Input: part model. Units: mm. Frame: model coordinates. A direction names the side the tool comes from. Give positions to 0.01 mm unless a question says otherwise; leave off trailing zeros. Order: outer loops, then holes, each group sorted by start corner. A loop starts at its lowest first (then second) coordinate and runs counter-clockwise, first axis right, second up. Notation, with made-up numbers: M 22,66 L 74,66 A25 cw 74,99 Z; hole C 73.25,-27.75 d8. An arc over 180 degrees is marked long. Use a Markdown table: item, result.
from build123d import *

# Parameters (mm, degrees)
SKETCH1_R           = 30
BOSS_EXTRUDE1_DEPTH = 25


with BuildPart() as part:
    # Sketch1 → Boss-Extrude1 (new body)
    with BuildSketch(Plane(origin=(0, 0, 0), x_dir=(1, 0, 0), z_dir=(0, 1, 0))):
        with BuildLine():
            Line((73, 18.485014011), (73, -18.485014011))
            ThreePointArc((73, -18.485014011), (98.171988791, -34.2), (108, -62.2))
            Line((108, -62.2), (108, -107))
            Line((108, -107), (63.2, -107))
            ThreePointArc((63.2, -107), (28.924287458, -91.048146036), (19.057555316, -54.552479005))
            ThreePointArc((19.057555316, -54.552479005), (15.86461811, -44.166949194), (5.59587046, -40.616329645))
            ThreePointArc((5.59587046, -40.616329645), (0, -41), (-5.59587046, -40.616329645))
            ThreePointArc((-5.59587046, -40.616329645), (-15.86461811, -44.166949194), (-19.057555316, -54.552479005))
            ThreePointArc((-19.057555316, -54.552479005), (-28.924287458, -91.048146036), (-63.2, -107))
            Line((-63.2, -107), (-108, -107))
            Line((-108, -107), (-108, -62.2))
            ThreePointArc((-108, -62.2), (-98.171988791, -34.2), (-73, -18.485014011))
            Line((-73, -18.485014011), (-73, 18.485014011))
            ThreePointArc((-73, 18.485014011), (-98.171988791, 34.2), (-108, 62.2))
            Line((-108, 62.2), (-108, 107))
            Line((-108, 107), (-63.2, 107))
            ThreePointArc((-63.2, 107), (-28.924287458, 91.048146036), (-19.057555316, 54.552479005))
            ThreePointArc((-19.057555316, 54.552479005), (-15.86461811, 44.166949194), (-5.59587046, 40.616329645))
            ThreePointArc((-5.59587046, 40.616329645), (0, 41), (5.59587046, 40.616329645))
            ThreePointArc((5.59587046, 40.616329645), (15.86461811, 44.166949194), (19.057555316, 54.552479005))
            ThreePointArc((19.057555316, 54.552479005), (28.924287458, 91.048146036), (63.2, 107))
            Line((63.2, 107), (108, 107))
            Line((108, 107), (108, 62.2))
            ThreePointArc((108, 62.2), (98.171988791, 34.2), (73, 18.485014011))
        make_face()
        with Locations(Location((0, 0, 0), (0, 0, 270))):
            Circle(SKETCH1_R, mode=Mode.SUBTRACT)
        with BuildLine():
            Line((86.274940548, 85.274940548), (86.274940548, 62.2))
            ThreePointArc((86.274940548, 62.2), (46.883553063, 45.883553063), (63.2, 85.274940548))
            Line((63.2, 85.274940548), (86.274940548, 85.274940548))
        make_face(mode=Mode.SUBTRACT)
        with BuildLine():
            Line((86.274940548, -85.274940548), (86.274940548, -62.2))
            ThreePointArc((86.274940548, -62.2), (46.883553063, -45.883553063), (63.2, -85.274940548))
            Line((63.2, -85.274940548), (86.274940548, -85.274940548))
        make_face(mode=Mode.SUBTRACT)
        with BuildLine():
            Line((-86.274940548, -85.274940548), (-86.274940548, -62.2))
            ThreePointArc((-86.274940548, -62.2), (-46.883553063, -45.883553063), (-63.2, -85.274940548))
            Line((-63.2, -85.274940548), (-86.274940548, -85.274940548))
        make_face(mode=Mode.SUBTRACT)
        with BuildLine():
            Line((-63.2, 85.274940548), (-86.274940548, 85.274940548))
            Line((-86.274940548, 85.274940548), (-86.274940548, 62.2))
            ThreePointArc((-86.274940548, 62.2), (-46.883553063, 45.883553063), (-63.2, 85.274940548))
        make_face(mode=Mode.SUBTRACT)
    extrude(amount=BOSS_EXTRUDE1_DEPTH)


solid = part.part
1) Cut plane A-A on x = 0. Return loops of the section in (y, z), and give its area (3 significant figures).
Response values:
| item | result |
|---|---|
| outline | M 0,-41 L 25,-41 L 25,-30 L 0,-30 Z; M 0,30 L 25,30 L 25,41 L 0,41 Z |
| area | 550 mm² |
2) Cut plane B-B on z = 0. Return loops of the section in (x, y).
Response values:
| item | result |
|---|---|
| outline | M -73,0 L -30,0 L -30,25 L -73,25 Z; M 30,0 L 73,0 L 73,25 L 30,25 Z |
3) Cut plane D-D on x = 76. Return loops of the section in (y, z), and give its area (3 significant figures).
Response values:
| item | result |
|---|---|
| outline | M 0,-107 L 25,-107 L 25,-85.27 L 0,-85.27 Z; M 0,-43 L 25,-43 L 25,-19.27 L 0,-19.27 Z; M 0,19.27 L 25,19.27 L 25,43 L 0,43 Z; M 0,85.27 L 25,85.27 L 25,107 L 0,107 Z |
| area | 2,270 mm² |
4) Mould query, pull axis X, two halves, no side actions, for faces 1 (the face through (98.435, 12.325, -34.532)), 2 (the face through (-108, 12, -84)), 3 (the face through (-86.275, 12, -74)), 4 (the face through (85, 12, -107)). Classes: released by +X, released by -X, zero draft, split by the parting line, or undercut.
Response values:
| item | result |
|---|---|
| face 1 | released by +X |
| face 2 | released by -X |
| face 3 | undercut |
| face 4 | zero draft |
5) Reachability of faces 5 (the face through (-73, 12, 0)), 6 (the face through (-86.275, 12, 74)), 7 (the face through (-108, 12, 85)) from +Z, -Z, +X, -X, +Y, -Y: full face, straight path, thin tool, end or side. Return the list, or none.
Response values:
| item | result |
|---|---|
| face 5 | -X, +Y, -Y |
| face 6 | +Y, -Y |
| face 7 | +Z, -Z, -X, +Y, -Y |
6) Cut plane C-C on z = -76. Return loops of the section in (x, y).
Response values:
| item | result |
|---|---|
| outline | M -108,0 L -86.27,0 L -86.27,25 L -108,25 Z; M -44.71,0 L -20.58,0 L -20.58,25 L -44.71,25 Z; M 20.58,0 L 44.71,0 L 44.71,25 L 20.58,25 Z; M 86.27,0 L 108,0 L 108,25 L 86.27,25 Z |
7) First-contact query: pin 1 Ø1 at (y, z) = (5.5, 49) entering from -X; pin 2 Ø1 at (x, y) = (46.5, 7.5) entering from +Z; pin 3 Ø2 at (x, z) = (-36.5, 34) entering from -Y; pin 4 Ø7.5 at (y, z) = (6.5, 1) entering from -X. Flat tips, straight axial feed; report the tip coordinate or a pass-through.
Response values:
| item | result |
|---|---|
| pin 1 | stops at x = -106.16 |
| pin 2 | stops at z = 103.97 |
| pin 3 | stops at y = 0 |
| pin 4 | stops at x = -73 |
8) Material intervals for line 1 (Z direction, x = -63.2, y = 16.75); line 2 (X direction, y = 13.5, z = -62.2); line 3 (Z direction, x = 55, y = 20.25), sorted ascending. Write a range as from..to.
Response values:
| item | result |
|---|---|
| line 1 | z = -107..-85.27, -39.13..39.13, 85.27..107 |
| line 2 | x = -108..-86.27, -40.13..-18.4, 18.4..40.13, 86.27..108 |
| line 3 | z = -106.24..-83.77, -40.63..40.63, 83.77..106.24 |
